Job drawing, mm, ordinate dimensions from the low corner. One solid piece. A direction names the side the tool comes from. Give positions to 0.01 mm unless a question says otherwise; leave off trailing zeros. Order: outer loops, then holes, each group sorted by start corner. A loop starts at its lowest first (then second) coordinate and runs counter-clockwise, first axis right, second up.
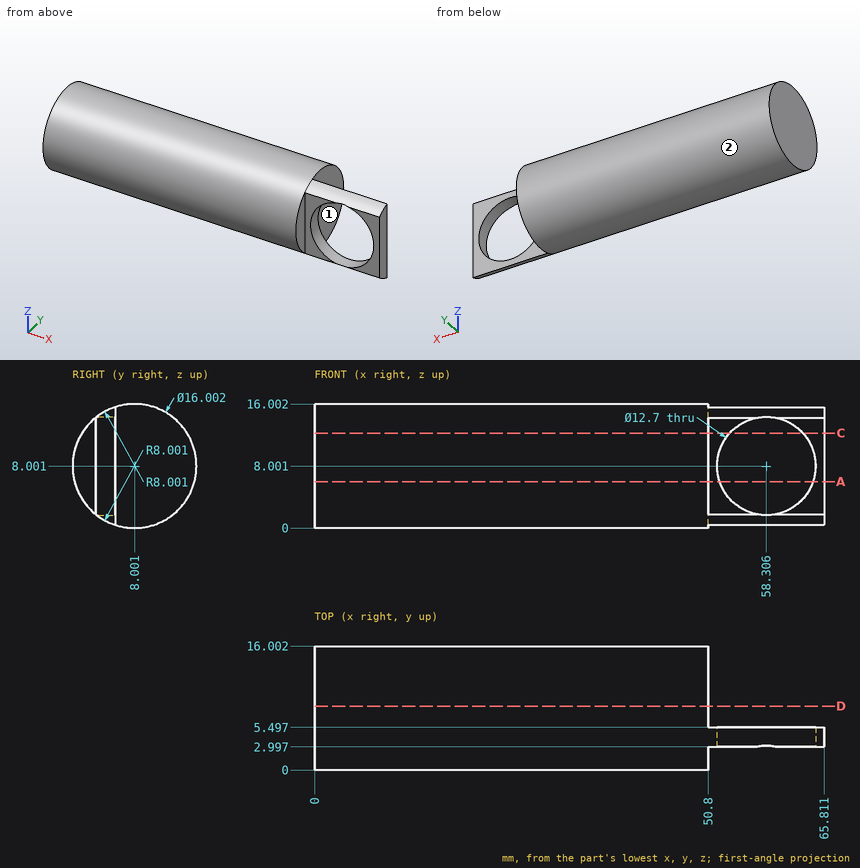
Item 1: Band-saw the part on C-C on z = 12.25. List the corners of the cut face in (x, y) (1 decimal).
Item 2: Which spindle directions (+Z, -Z, +X, -X, +Y, -Y) get a long thin tool onto all of the face, cutting with end or side? Do the marked faces 1 and 2. Say none if no direction does.
Item 3: Band-saw the part on D-D on y = 8.25. List the corners of the cut face in (x, z).
Item 4: Drill centre lines: probe 1 along X at (y, z) = (12.5, 3.5); probe 2 along Y at (x, z) = (53, 13.75); probe 3 along X at (y, z) = (5, 4.5) (1 decimal). Where is each one in solid material? Low to high.
Item 5: Band-saw the part on A-A on z = 6. List the corners of the cut face in (x, y) (1 decimal).
Item 6: Drop flat-ended pins along their axis: P1, Ø2, axis at x = 27.5, z = 10, coming from the +Y side; P2, Ø5, axis at x = 54, z = 9.5, coming from the -Y side; P3, Ø1, axis at x = 16, y = 9.5, coming from the +Z side. Give the stop position or say it passes through.
Working result:
1. outline: (0, 1.2) - (50.8, 1.2) - (50.8, 3) - (53.6, 3) - (53.6, 5.5) - (50.8, 5.5) - (50.8, 14.8) - (0, 14.8) - close; (63, 3) - (65.8, 3) - (65.8, 5.5) - (63, 5.5) - close
2. face 1: +Z, -Z, +X, +Y
2. face 2: +X, -X
3. outline: (0, 0) - (50.8, 0) - (50.8, 16) - (0, 16) - close
4. probe 1: x = 0 to 50.8
4. probe 2: y = 3 to 5.5
4. probe 3: x = 0 to 53, 63.6 to 65.8
5. outline: (0, 0.3) - (50.8, 0.3) - (50.8, 3) - (52.3, 3) - (52.3, 5.5) - (50.8, 5.5) - (50.8, 15.7) - (0, 15.7) - close; (64.3, 3) - (65.8, 3) - (65.8, 5.5) - (64.3, 5.5) - close
6. P1: stops at y = 15.94
6. P2: stops at y = 3
6. P3: stops at z = 15.94
